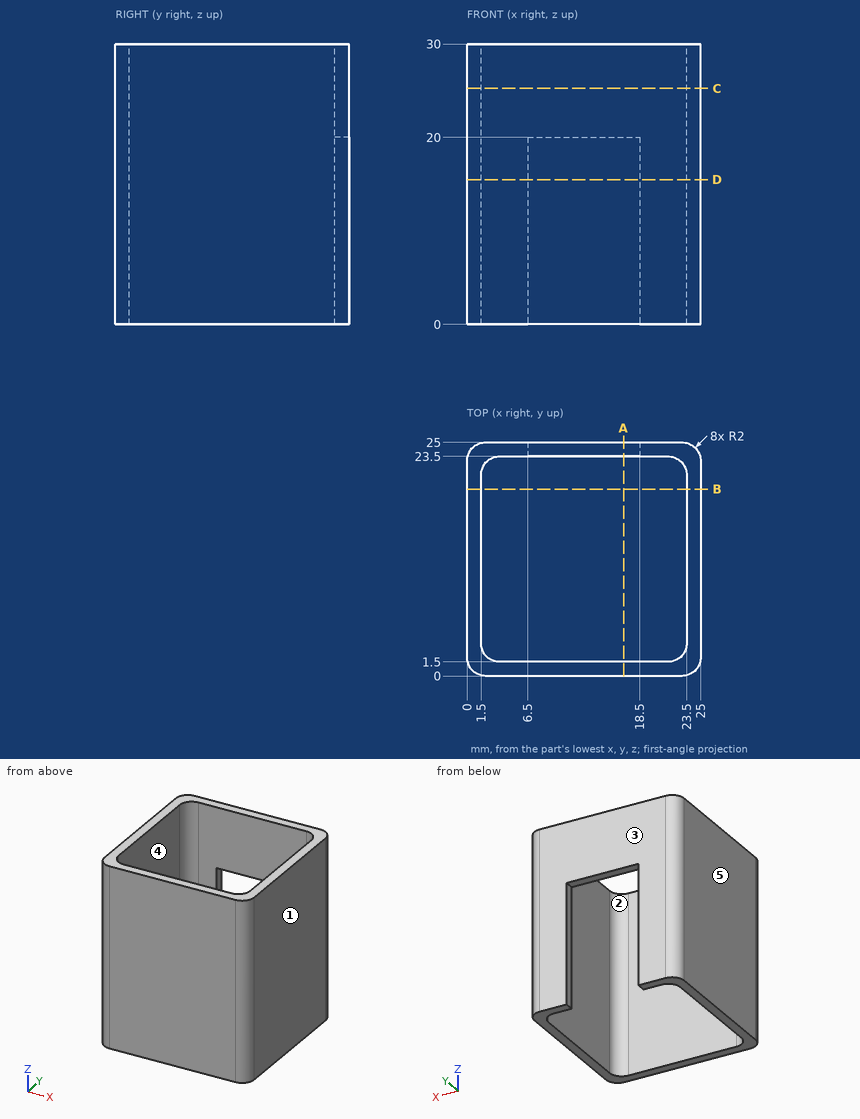
Input: dimensioned drawing with shaded views. Units: mm. Origin: part minimum x, y, z. A direction names the side the tool comes from. Give positions to 0.01 mm unless a question says otherwise; leave off trailing zeros. Loops run counter-clockwise (first coordinate to the right, second up) from the corner with the lowest first, then second, coordinate; pieces in that order, holes last. Notation, with made-up numbers: (45.25, 59.25) -> (50.25, 59.25) arc R21 ccw to (50.25, 63.25) -> close; hole circle Ø3 at (58, 3). An arc over 180 degrees is marked (long way). Use a Markdown table: item, result. Add a question column.
1) First-contact query: pin 1 (0.8 mm diameter, centred on y = 24, z = 10.5, fed in from +X); pin 2 (1.6 mm diameter, centred on x = 12.5, y = 24, fed in from -Z); pin 3 (1.2 mm diameter, centred on y = 24.5, z = 14.5, fed in from -X). Flat tips, straight axial feed; report the tip coordinate or a pass-through.
2) Line query: line 1 along Y through (x, z) = (19.25, 23); line 2 along Y through (x, z) = (14.75, 18). Output: solid intervals per line, ascending. Write a range as [from, to].
3) Pull-direction query (X, two-part tool) for the marked faces 1, 2 and 3; classes: +X half, -X half, draft (parallel to the pull), parting line (faces both ways), or undercut.
4) Section query B-B, the plane y = 20. Return the cut outline in (x, z), then the cut area to 3 significant figures.
5) Section query C-C, the plane z = 25.25. Return the cut outline in (x, y), then the cut area to 3 significant figures.
6) Section query A-A, the plane x = 16.75. Return the cut outline in (y, z), then the cut area to 3 significant figures.
7) Section query D-D, the plane z = 15.5. Return the cut outline in (x, y).
8) Reachability of the marked faces 4 and 5 from +Z, -Z, +X, -X, +Y, -Y: full face, straight path, thin tool, end or side. Return the list, or none.
Numbers:
| question | item | result |
|---|---|---|
| 1 | pin 1 | stops at x = 24.91 |
| 1 | pin 2 | stops at z = 20 |
| 1 | pin 3 | stops at x = 0.21 |
| 2 | line 1 | y = [0, 1.5], [23.5, 25] |
| 2 | line 2 | y = [0, 1.5] |
| 3 | face 1 | +X half |
| 3 | face 2 | undercut |
| 3 | face 3 | draft |
| 4 | outline | (0, 0) -> (1.5, 0) -> (1.5, 30) -> (0, 30) -> close; (23.5, 0) -> (25, 0) -> (25, 30) -> (23.5, 30) -> close |
| 4 | area | 90.0 mm2 |
| 5 | outline | (0, 2) arc R2 ccw to (2, 0) -> (23, 0) arc R2 ccw to (25, 2) -> (25, 23) arc R2 ccw to (23, 25) -> (2, 25) arc R2 ccw to (0, 23) -> close; hole (1.5, 3.5) arc R2 ccw to (3.5, 1.5) -> (21.5, 1.5) arc R2 ccw to (23.5, 3.5) -> (23.5, 21.5) arc R2 ccw to (21.5, 23.5) -> (3.5, 23.5) arc R2 ccw to (1.5, 21.5) -> close |
| 5 | area | 141 mm2 |
| 6 | outline | (0, 0) -> (1.5, 0) -> (1.5, 30) -> (0, 30) -> close; (23.5, 20) -> (25, 20) -> (25, 30) -> (23.5, 30) -> close |
| 6 | area | 60.0 mm2 |
| 7 | outline | (0, 2) arc R2 ccw to (2, 0) -> (23, 0) arc R2 ccw to (25, 2) -> (25, 23) arc R2 ccw to (23, 25) -> (18.5, 25) -> (18.5, 23.5) -> (21.5, 23.5) arc R2 cw to (23.5, 21.5) -> (23.5, 3.5) arc R2 cw to (21.5, 1.5) -> (3.5, 1.5) arc R2 cw to (1.5, 3.5) -> (1.5, 21.5) arc R2 cw to (3.5, 23.5) -> (6.5, 23.5) -> (6.5, 25) -> (2, 25) arc R2 ccw to (0, 23) -> close |
| 8 | face 4 | +Z, -Z |
| 8 | face 5 | +Z, -Z, -X, +Y, -Y |
